Verification items for the finished model (mm, model axes). A direction names the side the tool comes from. Give positions to 0.01 mm unless a question says otherwise; leave off trailing zeros. Order: outer loops, then holes, each group sorted by start corner. A loop starts at its lowest first (then second) coordinate and runs counter-clockwise, first axis right, second up. Notation, with made-up numbers: M -22,53 L -8,53 A16 ccw -8,69 Z; hole C 46.5,82 d1. An arc over 180 degrees is marked long. Answer as a JSON object with one key per item and string values.
```python
from build123d import *

# Parameters (mm, degrees)
SKETCH1_R                                      = 13.97
BOSS_EXTRUDE1_DEPTH                            = 6.35
CBORE_FOR_2_SOCKET_HEAD_CAP_SCREW1_D           = 2.2606
CBORE_FOR_2_SOCKET_HEAD_CAP_SCREW1_CBORE_D     = 4.7625
CBORE_FOR_2_SOCKET_HEAD_CAP_SCREW1_CBORE_DEPTH = 2.1844
CIRPATTERN1_COUNT                              = 3
CIRPATTERN2_COUNT                              = 3
CIRPATTERN3_COUNT                              = 3


with BuildPart() as part:
    # Sketch1 → Boss-Extrude1 (new body)
    with BuildSketch(Plane(origin=(0, 0, 0), x_dir=(1, 0, 0), z_dir=(0, 1, 0))):
        with Locations(Location((0, 0, 0), (0, 0, 270))):
            Circle(SKETCH1_R)
    extrude(amount=BOSS_EXTRUDE1_DEPTH)

    # CBORE for #2 Socket Head Cap Screw1 (through all)
    with Locations(Plane(origin=(0, 6.35, 0), x_dir=(1, 0, 0), z_dir=(0, 1, 0))):
        with Locations((7.363810019, -7.363810019)):
            cbore_for_2_socket_head_cap_screw1 = CounterBoreHole(CBORE_FOR_2_SOCKET_HEAD_CAP_SCREW1_D / 2, CBORE_FOR_2_SOCKET_HEAD_CAP_SCREW1_CBORE_D / 2, CBORE_FOR_2_SOCKET_HEAD_CAP_SCREW1_CBORE_DEPTH)

    # CirPattern1: CBORE for #2 Socket Head Cap Screw1 ×3 about axis
    cirpattern1_axis = Axis((0, 0, 0), (0, 1, 0))
    for i in range(1, CIRPATTERN1_COUNT):
        add(cbore_for_2_socket_head_cap_screw1.rotate(cirpattern1_axis, i * 360 / CIRPATTERN1_COUNT), mode=Mode.SUBTRACT)

    # Sketch10 → Tap Drill for #2-56 Tap2 (revolve, cut)
    with BuildSketch(Plane(origin=(7.977586831, 6.35, -6.693990167), x_dir=(0, 0, 1), z_dir=(1, 0, 0))):
        Polygon((0, 0), (0, 4.59816509), (0.889, 4.064), (0.889, 0), align=None)
    tap_drill_for_2_56_tap2 = revolve(axis=Axis((7.977586831, 12.7, -6.693990167), (0, -1, 0)), mode=Mode.SUBTRACT)

    # CirPattern2: Tap Drill for #2-56 Tap2 ×3 about axis
    cirpattern2_axis = Axis((0, 0, 0), (0, 1, 0))
    for i in range(1, CIRPATTERN2_COUNT):
        add(tap_drill_for_2_56_tap2.rotate(cirpattern2_axis, i * 360 / CIRPATTERN2_COUNT), mode=Mode.SUBTRACT)

    # Sketch15 → Tap Drill for #2-56 Tap1 (revolve, cut)
    with BuildSketch(Plane(origin=(-6.942501454, 3.105629072, 12.122812114), x_dir=(0.8677746681735182, 0, 0.4969578707258195), z_dir=(0, 1, 0))):
        Polygon((0, 0), (0, 7.095959572), (0.889, 6.35), (0.889, 0), align=None)
    tap_drill_for_2_56_tap1 = revolve(axis=Axis((-10.098183933, 3.105629072, 17.633181257), (0.4969578707258195, 0, -0.8677746681735182)), mode=Mode.SUBTRACT)

    # CirPattern3: Tap Drill for #2-56 Tap1 ×3 about axis
    cirpattern3_axis = Axis((0, 6.35, 0), (0, -1, 0))
    for i in range(1, CIRPATTERN3_COUNT):
        add(tap_drill_for_2_56_tap1.rotate(cirpattern3_axis, i * 360 / CIRPATTERN3_COUNT), mode=Mode.SUBTRACT)


solid = part.part
```
Q1. Gauge pin test, flat ends, axial feed: pin 1 Ø1.4 at (x, z) = (-9.79, -3.56) entering from +Y; pin 2 Ø1.1 at (x, z) = (1.81, 10.26) entering from +Y (3 decimals); pin 3 Ø3 at (y, z) = (2, 3) entering from +X; pin 4 Ø1.8 at (x, z) = (7.36, 7.36) entering from +Y. Record the tip position at first contact, or that the pin passes through.
Resolved:
{"pin 1": "stops at y = 2.18", "pin 2": "stops at y = 2.085", "pin 3": "stops at x = 13.89", "pin 4": "passes through"}
Q2. Tool access check on faces 4 (the face through (-3.42, 3.24, 6.11)), 5 (the face through (13.85, 3.13, -1.82)), 6 (the face through (-10, 4.166, 4)). Record the directions out of +Z, -Z, +X, -X, +Y, -Y that give a thin tool (end or side, any length) a straight path to the whole face; none if there is none.
Resolved:
{"face 4": "none", "face 5": "+Y, -Y", "face 6": "+Y"}
Q3. Material ranges on L1, parallel to X at y = 2.5, z = 10.5; L2, parallel to Z at x = 1.75, y = 5; L3, parallel to X at y = 5, z = -11.5, recorded low to high.
Resolved:
{"L1": "x = -9.21 to -6.76, -5.26 to 0.95, 2.66 to 9.21", "L2": "z = -13.86 to -12.24, -7.87 to 9.37, 11.14 to 13.86", "L3": "x = -7.93 to 0.8, 4.59 to 7.93"}
Q4. Release check for a two-part mould opening along Y. For faces 1 (the face through (-3.585, 3.243, -6.017)), 2 (the face through (3.794, 5.273, -7.947)), 3 (the face through (1.868, 1.845, 10.398)) record: +Y half, -Y half, draft (parallel to the pull), parting line (faces both ways), or undercut.
Resolved:
{"face 1": "undercut", "face 2": "draft", "face 3": "+Y half"}
Q5. Section check A-A on y = 4.75. Record the cut outline in (x, z) (1 decimal).
Resolved:
{"outline": "C 0,0 d27.9; hole C -10.1,2.7 d4.8; hole C -9.8,-3.6 d1.8; hole C 2.7,-10.1 d4.8; hole C 1.8,10.3 d1.8; hole C 7.4,7.4 d4.8; hole C 8,-6.7 d1.8"}
